Could you check a few things on this model? Use its own coordinates, in mm. Face numbers are marked on the shaded views. A direction names the side the tool comes from. Give positions to 0.01 mm unless a question says otherwise; leave off trailing zeros. Write each loop counter-clockwise with the first axis right and the second up, starting at its lowest first coordinate (ties: lowest second). Pieces come first, ordered by that corner, then holes. Notation, with made-up numbers: M 19,15.25 L 52,15.25 A22 ccw 52,25.25 Z; hole C 36,15 d2. An arc over 180 degrees is marked long. Answer as a JSON object with one key per item and string values. Group by question number.
```python
from build123d import *

# Parameters (mm, degrees)
SKETCH1_R           = 2.25
BOSS_EXTRUDE1_DEPTH = 10
SKETCH2_R           = 12
BOSS_EXTRUDE2_DEPTH = 30
SKETCH3_R           = 6
CUT_EXTRUDE1_DEPTH  = 48.16990566
CHAMFER1_SIZE       = 0.25
SKETCH4_R           = 3.5
CUT_EXTRUDE2_DEPTH  = 5


with BuildPart() as part:
    # Sketch1 → Boss-Extrude1 (new body)
    with BuildSketch(Plane.XY):
        with BuildLine():
            Line((-13.228756555, 15), (13.228756555, 15))
            ThreePointArc((13.228756555, 15), (20, 0), (13.228756555, -15))
            Line((13.228756555, -15), (-13.228756555, -15))
            ThreePointArc((-13.228756555, -15), (-20, 0), (-13.228756555, 15))
        make_face()
        with Locations((-16, 0)):
            Circle(SKETCH1_R, mode=Mode.SUBTRACT)
        with Locations((-11.313708499, 11.313708499)):
            Circle(SKETCH1_R, mode=Mode.SUBTRACT)
        with Locations((11.313708499, 11.313708499)):
            Circle(SKETCH1_R, mode=Mode.SUBTRACT)
        with Locations((16, 0)):
            Circle(SKETCH1_R, mode=Mode.SUBTRACT)
        with Locations((11.313708499, -11.313708499)):
            Circle(SKETCH1_R, mode=Mode.SUBTRACT)
        with Locations((-11.313708499, -11.313708499)):
            Circle(SKETCH1_R, mode=Mode.SUBTRACT)
    extrude(amount=BOSS_EXTRUDE1_DEPTH)

    # Sketch2 → Boss-Extrude2 (add)
    with BuildSketch(Plane.XY.offset(10)):
        Circle(SKETCH2_R)
    extrude(amount=BOSS_EXTRUDE2_DEPTH)

    # Sketch3 → Cut-Extrude1 (cut, through all)
    with BuildSketch(Plane.XY.offset(40)):
        Circle(SKETCH3_R)
    extrude(amount=-CUT_EXTRUDE1_DEPTH, mode=Mode.SUBTRACT)

    # Chamfer1
    chamfer1_edges = [part.edges().sort_by_distance(p)[0] for p in [
        (20, 0, 10),
        (0, 15, 10),
        (-12, 0, 40),
        (-20, 0, 10),
        (0, 15, 0),
        (20, 0, 0),
        (0, -15, 0),
        (-20, 0, 0),
        (0, -15, 10),
    ]]
    chamfer(chamfer1_edges, length=CHAMFER1_SIZE)

    # Sketch4 → Cut-Extrude2 (cut)
    with BuildSketch(Plane(origin=(0, 0, 0), x_dir=(-1, 0, 0), z_dir=(0, 0, -1))):
        with Locations((-11.313708499, 11.313708499)):
            Circle(SKETCH4_R)
        with Locations((11.313708499, 11.313708499)):
            Circle(SKETCH4_R)
        with Locations((16, 0)):
            Circle(SKETCH4_R)
        with Locations((11.313708499, -11.313708499)):
            Circle(SKETCH4_R)
        with Locations((-11.313708499, -11.313708499)):
            Circle(SKETCH4_R)
        with Locations((-16, 0)):
            Circle(SKETCH4_R)
    extrude(amount=-CUT_EXTRUDE2_DEPTH, mode=Mode.SUBTRACT)


solid = part.part
```
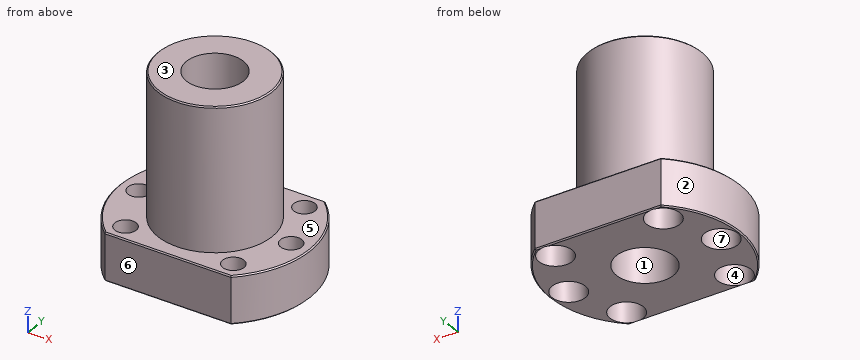
1) For the marked faces 5, 6 and 7, which set-ups out of +Z, -Z, +X, -X, +Y, -Y let a thin tool reach every point of the face, with its end or its side?
2) Please list where these lines run through material, in increasing order: line 1 along Y through (x, z) = (-16, 7.45); line 2 along X through (y, z) = (2, 7); line 3 along Z through (x, y) = (-13.5, 10). Write a range as from..to.
3) We'd pull the mould along X, two halves only. Please class the marked faces 1, 2, 3 and 4: released by +X, released by -X, zero draft, split by the parting line, or undercut.
4) If we section it at D-D, the plane z = 25.5: List the corners of the cut face in (x, y) for me.
5) If we section it at C-C, the plane z = 8: List the corners of the cut face in (x, y) for me.
6) If we section it at A-A, the plane x = 0: List the corners of the cut face in (y, z) for me, plus the area to 3 significant figures.
7) I'm going to push flat-ended pins straight in: pin 1 (15.5 mm diameter, centred on x = 0, y = 0, fed in from -Z); pin 2 (4 mm diameter, centred on x = -15.5, y = 6, fed in from +Z); pin 3 (10 mm diameter, centred on y = 4.5, z = 24.5, fed in from -X); pin 4 (3 mm diameter, centred on y = 9, z = 23, fed in from -X). Where does each tip first touch, or does it pass through?
8) If we section it at B-B, the plane y = 0: Give the number of separate pieces and of enclosed holes in the cut face, plus the area to 3 significant figures.
Taken from the geometry:
{
 "1": {"face 5": "+Z", "face 6": "+Z, -Z, +X, -X, -Y", "face 7": "-Z"},
 "2": {"line 1": "-12..-2.25, 2.25..12", "line 2": "-19.9..-17.03, -14.97..-5.66, 5.66..14.97, 17.03..19.9", "line 3": "5..10"},
 "3": {"face 1": "undercut", "face 2": "released by -X", "face 3": "zero draft", "face 4": "undercut"},
 "4": {"outline": "C 0,0 d24; hole C 0,0 d12"},
 "5": {"outline": "M -13.23,-15 L 13.23,-15 A20 ccw 13.23,15 L -13.23,15 A20 ccw Z; hole C -16,0 d4.5; hole C -11.31,-11.31 d4.5; hole C -11.31,11.31 d4.5; hole C 0,0 d12; hole C 11.31,-11.31 d4.5; hole C 11.31,11.31 d4.5; hole C 16,0 d4.5"},
 "6": {"outline": "M -15,0.25 L -14.75,0 L -6,0 L -6,40 L -11.75,40 L -12,39.75 L -12,10 L -14.75,10 L -15,9.75 Z; M 6,0 L 14.75,0 L 15,0.25 L 15,9.75 L 14.75,10 L 12,10 L 12,39.75 L 11.75,40 L 6,40 Z", "area": "540 mm²"},
 "7": {"pin 1": "z = 0", "pin 2": "z = 10", "pin 3": "x = -12", "pin 4": "x = -9.37"},
 "8": {"separate pieces": "4", "enclosed holes": "0", "area": "525 mm²"}
}
